For this review, take the finished solid that the model builds, in its own axes (mm). A direction names the side the tool comes from. Give positions to 0.01 mm unless a question says otherwise; leave off trailing zeros. Write each loop counter-clockwise with the first axis right and the second up, starting at its lowest first coordinate (ties: lowest second). Pieces come first, ordered by that corner, then holes. Notation, with made-up numbers: (44, 27) -> (48, 27) arc R38 ccw to (48, 66) -> close; hole circle Ø11 at (55.5, -12.5). An arc over 180 degrees is marked (long way). Write item = value, one per line.
```python
from build123d import *

# Parameters (mm, degrees)
BOSS_EXTRUDE1_DEPTH     = 27.94
CUT_EXTRUDE1_REACH      = 40.203
CUT_EXTRUDE1_END_RADIUS = 18.480456736
SKETCH2_R               = 2.54
SKETCH3_W               = 12.7
SKETCH3_H               = 0.8128
BOSS_EXTRUDE2_DEPTH     = 3.81
SKETCH4_W               = 12.7
SKETCH4_H               = 0.8128
BOSS_EXTRUDE3_DEPTH     = 3.81


with BuildPart() as part:
    # Sketch1 → Boss-Extrude1 (new body)
    with BuildSketch(Plane.XY):
        with BuildLine():
            Line((-25.065129767, -11.56137931), (2.874870233, -11.56137931))
            Line((2.874870233, -11.56137931), (2.874870233, -8.51337931))
            Line((2.874870233, -8.51337931), (-2.840129767, -8.51337931))
            Line((-2.840129767, -8.51337931), (-2.840129767, -4.44937931))
            ThreePointArc((-2.840129767, -4.44937931), (-11.095129767, -6.395560853), (-19.350129767, -4.44937931))
            Line((-19.350129767, -4.44937931), (-19.350129767, -8.51337931))
            Line((-19.350129767, -8.51337931), (-25.065129767, -8.51337931))
            Line((-25.065129767, -8.51337931), (-25.065129767, -11.56137931))
        make_face()
    extrude(amount=BOSS_EXTRUDE1_DEPTH)

    # Cut-Extrude1: up to this cylinder (the profile starts outside it)
    cut_extrude1_end = Plane(origin=(-11.095129767, 12.084895883, 13.97), z_dir=(0, 0, -1)) * Cylinder(CUT_EXTRUDE1_END_RADIUS, 118.366913471, mode=Mode.PRIVATE)
    # Sketch2 → Cut-Extrude1 (cut, up to the surface)
    with BuildSketch(Plane.XZ.offset(11.56137931), mode=Mode.PRIVATE) as cut_extrude1_sk1:
        with Locations(Location((-11.095129767, 13.97, 0), (0, 0, 270))):
            Circle(SKETCH2_R)
    cut_extrude1_tool1 = extrude(cut_extrude1_sk1.sketch, amount=-CUT_EXTRUDE1_REACH, mode=Mode.PRIVATE) - cut_extrude1_end
    add(cut_extrude1_tool1.solids().sort_by_distance((-11.09513, -11.561379, 13.97))[0], mode=Mode.SUBTRACT)

    # Sketch3 → Boss-Extrude2 (add)
    with BuildSketch(Plane(origin=(2.874870233, 0, 0), x_dir=(0, 0, -1), z_dir=(1, 0, 0))):
        with Locations((-13.97, -10.03737931)):
            Rectangle(SKETCH3_W, SKETCH3_H)
    extrude(amount=BOSS_EXTRUDE2_DEPTH)

    # Sketch4 → Boss-Extrude3 (add)
    with BuildSketch(Plane.ZY.offset(25.065129767)):
        with Locations((13.97, -10.03737931)):
            Rectangle(SKETCH4_W, SKETCH4_H)
    extrude(amount=BOSS_EXTRUDE3_DEPTH)


solid = part.part
```
(1) Tool access review of faces 1 (the face through (0, -8.513, 14)), 2 (the face through (5, -10, 7.62)), 3 (the face through (5, -10.444, 14)): name each direction out of +Z, -Z, +X, -X, +Y, -Y from which nothing blocks a thin tool from reaching the whole face with its end or side.
Answers below:
face_1 = +Z, -Z, +X, +Y
face_2 = -Z, +X, +Y, -Y
face_3 = +Z, -Z, +X, -Y
(2) Take a section at D-D (x = -12.5). Write out the cut boundary in (y, z).
Answers below:
outline = (-11.56, 0) -> (-6.34, 0) -> (-6.34, 11.85) -> (-11.56, 11.85) -> close; (-11.56, 16.09) -> (-6.34, 16.09) -> (-6.34, 27.94) -> (-11.56, 27.94) -> close
(3) To check wall thickness, follow probe 1 along X at (y, z) = (-8.3, 13.97); probe 2 along X at (y, z) = (-10.1, 13.97); probe 3 along X at (y, z) = (-10.75, 6.5). State the ranges of each line that lie inside material, in increasing order.
Answers below:
probe_1 = -19.35 to -13.64, -8.56 to -2.84
probe_2 = -28.88 to -13.64, -8.56 to 6.68
probe_3 = -25.07 to 2.87
(4) Take a section at B-B (y = -5.5). Write out the cut boundary in (x, z), plus the area to 3 significant figures.
Answers below:
outline = (-19.35, 0) -> (-16.78, 0) -> (-16.78, 27.94) -> (-19.35, 27.94) -> close; (-5.41, 0) -> (-2.84, 0) -> (-2.84, 27.94) -> (-5.41, 27.94) -> close
area = 144 mm^2
(5) Take a section at C-C (z = 22). Write out the cut boundary in (x, y), plus the area to 3 significant figures.
Answers below:
outline = (-25.07, -11.56) -> (2.87, -11.56) -> (2.87, -8.51) -> (-2.84, -8.51) -> (-2.84, -4.45) arc R18.48 cw to (-19.35, -4.45) -> (-19.35, -8.51) -> (-25.07, -8.51) -> close
area = 131 mm^2
(6) Take a section at A-A (z = 13.97). Write out the cut boundary in (x, y).
Answers below:
outline = (-28.88, -10.44) -> (-25.07, -10.44) -> (-25.07, -11.56) -> (-13.64, -11.56) -> (-13.64, -6.22) arc R18.48 cw to (-19.35, -4.45) -> (-19.35, -8.51) -> (-25.07, -8.51) -> (-25.07, -9.63) -> (-28.88, -9.63) -> close; (-8.56, -11.56) -> (2.87, -11.56) -> (2.87, -10.44) -> (6.68, -10.44) -> (6.68, -9.63) -> (2.87, -9.63) -> (2.87, -8.51) -> (-2.84, -8.51) -> (-2.84, -4.45) arc R18.48 cw to (-8.56, -6.22) -> close
(7) For pin 1 (1.2 mm diameter, centred on y = -6.5, z = 14, fed in from -X); pin 2 (1.9 mm diameter, centred on x = 5.5, z = 13, fed in from -Y); pin 3 (4 mm diameter, centred on x = 4.5, z = 16.5, fed in from +Y); pin 4 (6.5 mm diameter, centred on x = -11.1, z = 13.97, fed in from -Y), all flat-tipped, find the tip position at first contact; note any pin that passes through.
Answers below:
pin_1 = -19.35
pin_2 = -10.44
pin_3 = -8.51
pin_4 = -11.56
